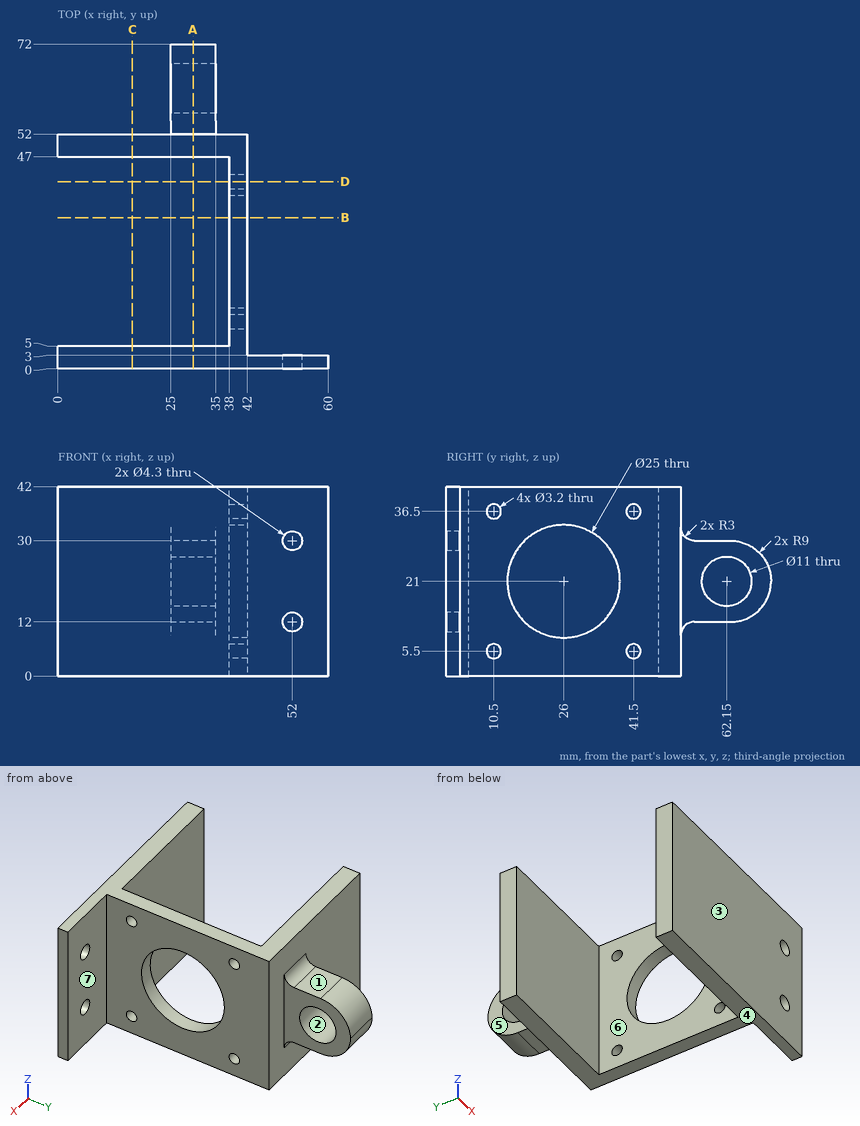
Drawing for the job (mm, zero at the part's lowest x, y, z). A direction names the side the tool comes from. Coordinates: 2 decimals unless noted, no trailing zeros. Order: outer loops, then holes, each group sorted by start corner. A loop starts at its lowest first (then second) coordinate and runs counter-clockwise, first axis right, second up.
Item 1: Two-plate mould, pull along Z, no slides. Class the marked faces 1, 2 and 3: +Z half, -Z half, draft (parallel to the pull), parting line (faces both ways), or undercut.
Check sheet entries:
face 1: +Z half
face 2: undercut
face 3: draft
Item 2: Drill centre lines: L1, parallel to Y at x = 41.15, z = 36.5; L2, parallel to Y at x = 36.5, z = 16; L3, parallel to X at y = 1, z = 12. Where is each one in solid material? Low to high.
Check sheet entries:
L1: y = 0 to 8.9, 12.1 to 39.9, 43.1 to 52
L2: y = 0 to 5, 47 to 52
L3: x = 0 to 49.85, 54.15 to 60
Item 3: Pin check, flat tips, straight feed: pin 1 Ø2.5 at (x, y) = (28, 57.5) entering from +Z; pin 2 Ø10 at (x, z) = (9.5, 13.5) entering from +Y; pin 3 Ø16 at (y, z) = (66.5, 15) entering from -X; pin 4 Ø8 at (x, y) = (42.5, 61.5) entering from +Z. Stop position of each tip, or through.
Check sheet entries:
pin 1: stops at z = 30
pin 2: stops at y = 52
pin 3: stops at x = 25
pin 4: passes through
Item 4: 3-axis set-ups, long thin cutter, end or side, ignore diameter. For the marked faces 4, 5, 6 and 7: which of +Z, -Z, +X, -X, +Y, -Y reach the whole face in a straight line?
Check sheet entries:
face 4: -Z, +X, -X, +Y, -Y
face 5: +Z, -Z, -X, +Y
face 6: +Z, -Z, -X
face 7: +Z, -Z, +X, +Y
Item 5: Band-saw the part on B-B on y = 33.5. List the corners of the cut face in (x, z), plus the area to 3 significant figures.
Check sheet entries:
outline: (38, 0) - (42, 0) - (42, 11) - (38, 11) - close; (38, 31) - (42, 31) - (42, 42) - (38, 42) - close
area: 88.0 mm2
Item 6: Band-saw the part on C-C on x = 16.5. List the corners of the cut face in (y, z), plus the area to 3 significant figures.
Check sheet entries:
outline: (0, 0) - (5, 0) - (5, 42) - (0, 42) - close; (47, 0) - (52, 0) - (52, 42) - (47, 42) - close
area: 420 mm2
Item 7: Band-saw the part on A-A on x = 30. Give the number of separate pieces and of enclosed holes in the cut face, plus the area to 3 significant figures.
Check sheet entries:
separate pieces: 2
enclosed holes: 1
area: 654 mm2
Item 8: Band-saw the part on D-D on y = 41.5. List the corners of the cut face in (x, z).
Check sheet entries:
outline: (38, 0) - (42, 0) - (42, 3.9) - (38, 3.9) - close; (38, 7.1) - (42, 7.1) - (42, 34.9) - (38, 34.9) - close; (38, 38.1) - (42, 38.1) - (42, 42) - (38, 42) - close
